Read the model definition and answer for the solid it produces. Units are mm, in the model's axes. A direction names the side the tool comes from. Round coordinates to 2 decimals unless told otherwise and drop trailing zeros. Write each loop counter-clockwise with the first axis right and the second up, starting at its lowest first coordinate (ties: lowest second). Pieces come first, ordered by that corner, then holes.
from build123d import *

# Parameters (mm, degrees)
F0_W      = 126
F0_H      = 56
F1_DEPTH  = 108
F2_T      = -1.8
F3_R      = 1.8
F4_R      = 2.5
F5_DEPTH  = 25
F6_W      = 124.2
F6_H      = 30
F7_DEPTH  = 120
F8_R      = 3.6
F10_DEPTH = 56
F11_R     = 2
F12_DEPTH = 25
F13_R     = 2
F14_DEPTH = 25


with BuildPart() as f1:
    # F0 (on Front) → F1 (new body)
    with BuildSketch(Plane.XZ):
        Rectangle(F0_W, F0_H)
    extrude(amount=F1_DEPTH)

    # F2
    f2_openings = [f1.faces().sort_by_distance(p)[0] for p in [
        (0, -108, 0),
    ]]
    offset(amount=F2_T, openings=f2_openings)

    # F3
    f3_edges = [f1.edges().sort_by_distance(p)[0] for p in [
        (-61.2, -1.8, 0),
        (-61.2, -54.9, -26.2),
        (0, -1.8, -26.2),
        (0, -1.8, 26.2),
        (-61.2, -54.9, 26.2),
        (61.2, -1.8, 0),
        (61.2, -54.9, 26.2),
        (61.2, -54.9, -26.2),
    ]]
    fillet(f3_edges, radius=F3_R)

    # F4 (on face) → F5 (cut)
    with BuildSketch(Plane(origin=(-63, 0, 0), x_dir=(0, -1, 0), z_dir=(-1, 0, 0))):
        with BuildLine():
            ThreePointArc((36, 0), (30, 6), (24, 0))
            Line((24, 0), (30, 0))
            Line((30, 0), (30, -6))
            ThreePointArc((30, -6), (34.2426406871, -4.2426406871), (36, 0))
        make_face()
        with BuildLine():
            ThreePointArc((32.5, -18), (31.767766953, -16.232233047), (30, -15.5))
            ThreePointArc((30, -15.5), (28.232233047, -19.767766953), (32.5, -18))
        make_face()
        with BuildLine():
            Line((30, 0), (24, 0))
            ThreePointArc((24, 0), (25.7573593129, -4.2426406871), (30, -6))
            Line((30, -6), (30, 0))
        make_face()
        with Locations((30, 18)):
            Circle(F4_R)
    extrude(amount=-F5_DEPTH, mode=Mode.SUBTRACT)

    # F6 (on face) → F7 (cut)
    with BuildSketch(Plane(origin=(0, 0, 0), x_dir=(-1, 0, 0), z_dir=(0, 1, 0))):
        with Locations((-0.9, 0)):
            Rectangle(F6_W, F6_H)
    extrude(amount=-F7_DEPTH, mode=Mode.SUBTRACT)

    # F8
    f8_edges = [f1.edges().sort_by_distance(p)[0] for p in [
        (0, 0, -28),
        (63, -54, -28),
        (63, 0, -21.5),
        (63, 0, 21.5),
        (63, -54, 28),
        (0, 0, 28),
        (-63, -54, 28),
        (-63, -54, -28),
    ]]
    fillet(f8_edges, radius=F8_R)

    # F9 (on face) → F10 (cut)
    with BuildSketch(Plane.XY.offset(28)):
        with BuildLine():
            Line((20.7846096908, -108), (5.18, -108))
            Line((5.18, -108), (0, -108))
            Line((0, -108), (0, -96))
            ThreePointArc((0, -96), (-16.9705627485, -136.9705627485), (24, -120))
            ThreePointArc((24, -120), (23.1822198309, -113.7883429175), (20.7846096908, -108))
        make_face()
        with BuildLine():
            Line((5.18, -96.5656747484), (5.18, -108))
            Line((5.18, -108), (20.7846096908, -108))
            ThreePointArc((20.7846096908, -108), (14.1854216571, -100.6409242883), (5.18, -96.5656747484))
        make_face()
        with BuildLine():
            Line((0, -108), (5.18, -108))
            Line((5.18, -108), (5.18, -96.5656747484))
            ThreePointArc((5.18, -96.5656747484), (2.6053976626, -96.1418378114), (0, -96))
            Line((0, -96), (0, -108))
        make_face()
        with BuildLine():
            ThreePointArc((10.28, -40.23), (1.5737554159, -36.6237554159), (5.18, -45.33))
            ThreePointArc((5.18, -45.33), (8.7862445841, -43.8362445841), (10.28, -40.23))
        make_face()
    extrude(amount=-F10_DEPTH, mode=Mode.SUBTRACT)

    # F11 (on face) → F12 (cut)
    with BuildSketch(Plane.YZ.offset(63)):
        with BuildLine():
            ThreePointArc((-97.5, 19.7), (-99.5, 21.7), (-101.5, 19.7))
            Line((-101.5, 19.7), (-99.5, 19.7))
            Line((-99.5, 19.7), (-97.5, 19.7))
        make_face()
        with BuildLine():
            ThreePointArc((-6.5, 19.7), (-8.5, 21.7), (-10.5, 19.7))
            ThreePointArc((-10.5, 19.7), (-8.5, 17.7), (-6.5, 19.7))
        make_face()
        with BuildLine():
            Line((-99.5, 19.7), (-101.5, 19.7))
            ThreePointArc((-101.5, 19.7), (-99.5, 17.7), (-97.5, 19.7))
            Line((-97.5, 19.7), (-99.5, 19.7))
        make_face()
        with Locations((-8.5, -19.7)):
            Circle(F11_R)
        with Locations((-99.5, -19.7)):
            Circle(F11_R)
    extrude(amount=-F12_DEPTH, mode=Mode.SUBTRACT)

    # F13 (on face) → F14 (cut)
    with BuildSketch(Plane(origin=(0, 0, 0), x_dir=(-1, 0, 0), z_dir=(0, 1, 0))):
        with BuildLine():
            ThreePointArc((-49.9, 19.7), (-51.9, 21.7), (-53.9, 19.7))
            Line((-53.9, 19.7), (-51.9, 19.7))
            Line((-51.9, 19.7), (-49.9, 19.7))
        make_face()
        with BuildLine():
            ThreePointArc((56.1, 19.7), (54.1, 21.7), (52.1, 19.7))
            ThreePointArc((52.1, 19.7), (54.1, 17.7), (56.1, 19.7))
        make_face()
        with BuildLine():
            Line((-51.9, 19.7), (-53.9, 19.7))
            ThreePointArc((-53.9, 19.7), (-51.9, 17.7), (-49.9, 19.7))
            Line((-49.9, 19.7), (-51.9, 19.7))
        make_face()
        with Locations((54.1, -19.7)):
            Circle(F13_R)
        with Locations((-51.9, -19.7)):
            Circle(F13_R)
    extrude(amount=-F14_DEPTH, mode=Mode.SUBTRACT)


solid = f1.part
Q1. Section C-C (x = 17.5) is taken. Determine the outline of the cut face in (y, z), then the cut area to 3 significant figures.
Verdict:
outline: (-103.58, -28) - (-3.6, -28) arc R3.6 ccw to (0, -24.4) - (0, -15) - (-1.8, -15) - (-1.8, -24.4) arc R1.8 cw to (-3.6, -26.2) - (-103.58, -26.2) - close; (-103.58, 26.2) - (-3.6, 26.2) arc R1.8 cw to (-1.8, 24.4) - (-1.8, 15) - (0, 15) - (0, 24.4) arc R3.6 ccw to (-3.6, 28) - (-103.58, 28) - close
area: 409 mm2
Q2. Section A-A (x = 51.9) is taken. Determine the outline of the cut face in (y, z).
Verdict:
outline: (-108, -28) - (-3.6, -28) arc R3.6 ccw to (0, -24.4) - (0, -21.7) - (-1.8, -21.7) - (-1.8, -24.4) arc R1.8 cw to (-3.6, -26.2) - (-108, -26.2) - close; (-108, 26.2) - (-3.6, 26.2) arc R1.8 cw to (-1.8, 24.4) - (-1.8, 21.7) - (0, 21.7) - (0, 24.4) arc R3.6 ccw to (-3.6, 28) - (-108, 28) - close; (-1.8, -17.7) - (0, -17.7) - (0, -15) - (-1.8, -15) - close; (-1.8, 15) - (0, 15) - (0, 17.7) - (-1.8, 17.7) - close
Q3. Section D-D (z = 2) is taken. Determine the outline of the cut face in (x, y).
Verdict:
outline: (-63, -108) - (-61.2, -108) - (-61.2, -35.66) - (-63, -35.66) - close; (-63, -24.34) - (-61.2, -24.34) - (-61.2, 0) - (-63, 0) - close
Q4. A flat-ended cylindrical pin translates along its axis: pin 1 Ø10.5 at (x, z) = (-25, -18.5) entering from -Y. Find the tip coordinate at first contact, or state that the pin passes through.
Verdict:
pin 1: stops at y = -1.8
Q5. Section B-B (y = -8.5) is taken. Determine the outline of the cut face in (x, z).
Verdict:
outline: (-63, -24.4) arc R3.6 ccw to (-59.4, -28) - (59.4, -28) arc R3.6 ccw to (63, -24.4) - (63, -21.7) - (61.2, -21.7) - (61.2, -24.4) arc R1.8 cw to (59.4, -26.2) - (-59.4, -26.2) arc R1.8 cw to (-61.2, -24.4) - (-61.2, 24.4) arc R1.8 cw to (-59.4, 26.2) - (59.4, 26.2) arc R1.8 cw to (61.2, 24.4) - (61.2, 21.7) - (63, 21.7) - (63, 24.4) arc R3.6 ccw to (59.4, 28) - (-59.4, 28) arc R3.6 ccw to (-63, 24.4) - close; (61.2, -17.7) - (63, -17.7) - (63, -15) - (61.2, -15) - close; (61.2, 15) - (63, 15) - (63, 17.7) - (61.2, 17.7) - close
Q6. Which of the six approach directions +Z, -Z, +X, -X, +Y, -Y give full straight-line access (tool end or side, diameter ignored) to faces 1 (the flat face through (61.2, -55, -20)), 2 (the flat face through (-63, -53, 0)), 3 (the cylindrical face through (62.113, -97.592, -19.099))?
Verdict:
face 1: -Y
face 2: +Z, -Z, -X, +Y, -Y
face 3: +X
Q7. Straight lines are drawn through the part: probe 1 along Z at (x, y) = (51.9, -1.05); probe 2 along X at (y, z) = (-20, -19); probe 3 along Z at (x, y) = (35, -102.5). For each, find the intervals that lie inside material, in ascending order.
Verdict:
probe 1: z = -26.94 to -21.7, -17.7 to -15, 15 to 17.7, 21.7 to 26.94
probe 2: x = -63 to -61.2, 61.2 to 63
probe 3: z = -28 to -26.2, 26.2 to 28
Q8. Determine the mould class of faces 4 (the flat face through (-1, -55, -26.2)), 5 (the cylindrical face through (61.92, -56.53, 26.97)), 6 (the cylindrical face through (-61.97, -54.76, 26.92)) for opening direction X: pulls with the +X half, pulls with the -X half, needs draft (parallel to the pull), parting line crosses it, or undercut.
Verdict:
face 4: undercut
face 5: pulls with the +X half
face 6: pulls with the -X half
